```python
from build123d import *

# Parameters (mm, degrees)
F1_DEPTH = 4
F2_R     = 1


with BuildPart() as f1:
    # F0 (on Top) → F1 (new body)
    with BuildSketch(Plane.XY):
        with BuildLine():
            Line((45, 0), (-45, 0))
            Line((-45, 0), (-45, -10))
            ThreePointArc((-45, -10), (-42.071068, -17.071068), (-35, -20))
            Line((-35, -20), (35, -20))
            ThreePointArc((35, -20), (42.071068, -17.071068), (45, -10))
            Line((45, -10), (45, 0))
        make_face()
    extrude(amount=F1_DEPTH)

    # F2
    f2_edges = [f1.edges().sort_by_distance(p)[0] for p in [
        (-45, -5, 4),
        (-42.071068, -17.071068, 0),
    ]]
    fillet(f2_edges, radius=F2_R)


solid = f1.part
```
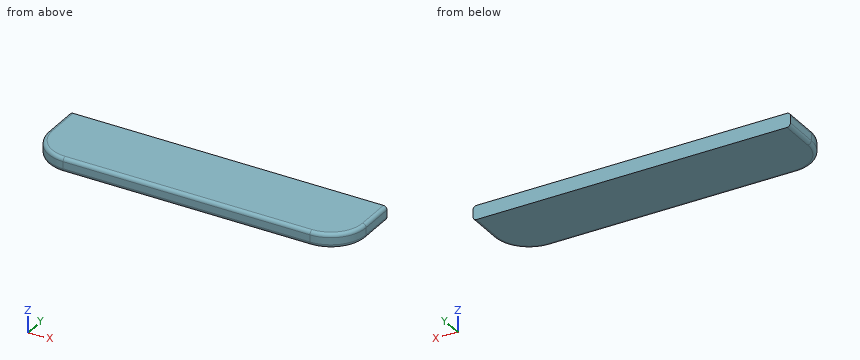
The model under review builds one solid part; all positions refer to its coordinate system, in mm. Give positions to 0.01 mm unless a question says otherwise; leave off trailing zeros. Write each loop counter-clockwise with the first axis right and the second up, starting at its lowest first coordinate (ties: lowest second). Pieces come first, ordered by that corner, then holes. Notation, with made-up numbers: (29.5, -7) -> (53.5, -7) arc R19 cw to (53.5, 9) -> close; hole circle Ø11 at (23, 62.25). An arc over 180 degrees is marked (long way). Put each result on its own line as item: value.
(1) We need section A-A, the plane z = 1.85. Give the boundary of the cut face in (x, y), and give its area (3 significant figures).
Results are:
outline: (-45, -10) arc R10 ccw to (-35, -20) -> (35, -20) arc R10 ccw to (45, -10) -> (45, 0) -> (-45, 0) -> close
area: 1,760 mm²
(2) For pin 1 Ø2 at (y, z) = (-18, 3.5) entering from -X; pin 2 Ø1.5 at (y, z) = (-12, 2.5) entering from +X, all flat-tipped, find the tip position at first contact; note any pin that passes through.
Results are:
pin 1: x = -42.07
pin 2: x = 44.92
(3) To check wall thickness, follow probe 1 along Y at (x, z) = (22.5, 3.6); probe 2 along X at (y, z) = (-17, 0.9); probe 3 along Y at (x, z) = (2, 3.25). State the ranges of each line that lie inside material, in increasing order. Write a range as from..to.
Results are:
probe 1: -19.8..0
probe 2: -42.13..42.13
probe 3: -19.97..0
